```python
from build123d import *

# Parameters (mm, degrees)
EXTRUSION1_DEPTH = 254
ESQUISSE2_R      = 1.5
EXTRUSION2_DEPTH = 186
ESQUISSE3_R      = 1.5
EXTRUSION3_DEPTH = 186


with BuildPart() as part:
    # Esquisse1 → Extrusion1 (new body)
    with BuildSketch(Plane.XY):
        Polygon((-21.235396624, -5.627388535), (-21.235396624, -20.627388535), (-6.235396624, -20.627388535), (-6.235396624, -19.127388535), (-19.735396624, -19.127388535), (-19.735396624, -5.627388535), align=None)
    extrude(amount=EXTRUSION1_DEPTH)

    # Esquisse2 → Extrusion2 (cut)
    with BuildSketch(Plane(origin=(0, -19.127388535, 0), x_dir=(-1, 0, 0), z_dir=(0, 1, 0))):
        with Locations(Location((13.735396624, 7, 0), (0, 0, 90))):
            Circle(ESQUISSE2_R)
        with Locations(Location((13.235396624, 250, 0), (0, 0, 90))):
            Circle(ESQUISSE2_R)
        with Locations(Location((13.235396624, 240, 0), (0, 0, 90))):
            Circle(ESQUISSE2_R)
    extrude(amount=-EXTRUSION2_DEPTH, mode=Mode.SUBTRACT)

    # Esquisse3 → Extrusion3 (cut)
    with BuildSketch(Plane(origin=(-19.735396624, 0, 0), x_dir=(0, 0, -1), z_dir=(1, 0, 0))):
        with Locations((-6, -13.127388535)):
            Circle(ESQUISSE3_R)
        with Locations((-246.5, -13.127388535)):
            Circle(ESQUISSE3_R)
    extrude(amount=-EXTRUSION3_DEPTH, mode=Mode.SUBTRACT)


solid = part.part
```
CAD build for the part. Positions are in the model's coordinates, mm. A direction names the side the tool comes from. Round coordinates to 2 decimals unless told otherwise and drop trailing zeros. Order: outer loops, then holes, each group sorted by start corner. A loop starts at its lowest first (then second) coordinate and runs counter-clockwise, first axis right, second up.
Item 1: Pin check, flat tips, straight feed: pin 1 (1 mm diameter, centred on x = -18, y = -13.5, fed in from +Z); pin 2 (1.5 mm diameter, centred on y = -17, z = 199.5, fed in from +X); pin 3 (1.5 mm diameter, centred on x = -10, z = 73.5, fed in from +Y). Stop position of each tip, or through.
Item 2: Probe line 1 along X through (y, z) = (-19.7, 250); line 2 along X through (y, z) = (-19.6, 7); line 3 along X through (y, z) = (-13.75, 54). List the from-to ranges inside material, lowest first.
Item 3: Saw through at A-A on z = 82.5. Write the cut outline in (x, y), then the cut area to 4 significant figures.
Item 4: Tool access for faces 1 (the face through (-14, -20.627, 125)), 2 (the face through (-13, -19.127, 125)): list every direction of +Z, -Z, +X, -X, +Y, -Y with a clear straight run to the whole face (end or side of a thin tool).
Item 5: Saw through at B-B on y = -9. Write the cut outline in (x, z), then the cut area to 3 significant figures.
Reported:
1. pin 1: passes through
1. pin 2: stops at x = -19.74
1. pin 3: stops at y = -19.13
2. line 1: x = -21.24 to -14.74, -11.74 to -6.24
2. line 2: x = -21.24 to -15.24, -12.24 to -6.24
2. line 3: x = -21.24 to -19.74
3. outline: (-21.24, -20.63) - (-6.24, -20.63) - (-6.24, -19.13) - (-19.74, -19.13) - (-19.74, -5.63) - (-21.24, -5.63) - close
3. area: 42.75 mm2
4. face 1: +Z, -Z, +X, -X, -Y
4. face 2: +Z, -Z, +X, +Y
5. outline: (-21.24, 0) - (-19.74, 0) - (-19.74, 254) - (-21.24, 254) - close
5. area: 381 mm2
